Read the model definition and answer for the solid it produces. Units are mm, in the model's axes. Face numbers are marked on the shaded views. A direction names the side the tool comes from. Coordinates: 2 decimals unless noted, no trailing zeros. Write each loop counter-clockwise with the first axis right and the second up, starting at its lowest first coordinate (ties: lowest second). Pieces come first, ordered by that corner, then holes. Notation, with made-up numbers: (52.5, -37.75) - (64.5, -37.75) arc R25 cw to (64.5, -15.75) - close; hole circle Ø1 at (21, -28.75). An arc over 180 degrees is marked (long way). Use a Markdown table: item, result.
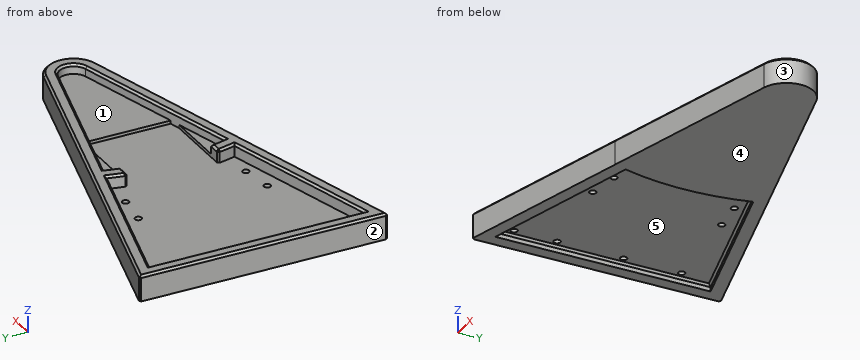
from build123d import *
from OCP.BRepFilletAPI import BRepFilletAPI_MakeChamfer

# Parameters (mm, degrees)
BOSS_EXTRUDE1_DEPTH     = 6
BOSS_EXTRUDE2_START     = 6
BOSS_EXTRUDE2_DEPTH     = 6
BOSS_EXTRUDE3_DEPTH     = 1.5
CUT_EXTRUDE3_DEPTH      = 6
CHAMFER1_SIZE           = 0.858848527
CHAMFER1_SIZE_2         = 1
CHAMFER2_SIZE           = 1
CHAMFER3_SIZE           = 1
CHAMFER3_SIZE2          = 0.816496581
CUT_EXTRUDE4_DEPTH      = 3
CHAMFER4_SIZE           = 1
CUT_EXTRUDE5_DEPTH      = 178.282114668
CUT_EXTRUDE5_DEPTH_BACK = 178.282114668
SKETCH8_R               = 1.55


with BuildPart() as part:
    # Sketch3 → Boss-Extrude1 (new body)
    with BuildSketch(Plane.XY):
        with BuildLine():
            Line((3.263957589, 12.181255556), (-167.389036276, 57.907587448))
            Line((-167.389036276, 57.907587448), (-167.389036276, -57.907587448))
            Line((-167.389036276, -57.907587448), (-83.597968128, -35.455838404))
            Line((-83.597968128, -35.455838404), (3.263957589, -12.181255556))
            ThreePointArc((3.263957589, -12.181255556), (12.610963724, 0), (3.263957589, 12.181255556))
        make_face()
    extrude(amount=BOSS_EXTRUDE1_DEPTH)

    # Sketch3<3> → Boss-Extrude2 (add)
    with BuildSketch(Plane.XY.offset(BOSS_EXTRUDE2_START)):
        with BuildLine():
            ThreePointArc((3.263957589, -12.181255556), (12.610963724, 0), (3.263957589, 12.181255556))
            Line((3.263957589, 12.181255556), (-167.389036276, 57.907587448))
            Line((-167.389036276, 57.907587448), (-167.389036276, -57.907587448))
            Line((-167.389036276, -57.907587448), (-83.597968128, -35.455838404))
            Line((-83.597968128, -35.455838404), (3.263957589, -12.181255556))
        make_face()
        with BuildLine():
            Line((1.711043318, -6.385700598), (-79.486479098, -28.142511157))
            ThreePointArc((-79.486479098, -28.142511157), (-83.143036276, 0), (-79.486479098, 28.142511157))
            Line((-79.486479098, 28.142511157), (1.711043318, 6.385700598))
            ThreePointArc((1.711043318, 6.385700598), (6.610963724, 0), (1.711043318, -6.385700598))
        make_face(mode=Mode.SUBTRACT)
        with BuildLine():
            Line((-85.282065581, -29.695433875), (-161.389036276, -50.088235211))
            Line((-161.389036276, -50.088235211), (-161.389036276, 50.088235211))
            Line((-161.389036276, 50.088235211), (-85.282065581, 29.695433875))
            ThreePointArc((-85.282065581, 29.695433875), (-89.143036276, 0), (-85.282065581, -29.695433875))
        make_face(mode=Mode.SUBTRACT)
    extrude(amount=BOSS_EXTRUDE2_DEPTH)

    # Sketch4 → Boss-Extrude3 (add)
    with BuildSketch(Plane.XY.offset(6)):
        with BuildLine():
            ThreePointArc((-79.486479098, 28.142511157), (-80.363791639, 24.584864194), (-81.12226241, 21))
            Line((-81.12226241, 21), (-52.830264568, 21))
            Line((-52.830264568, 21), (-79.486479098, 28.142511157))
        make_face()
        with BuildLine():
            Line((-79.486479098, -28.142511157), (-52.830264568, -21))
            Line((-52.830264568, -21), (-81.12226241, -21))
            ThreePointArc((-81.12226241, -21), (-80.363791639, -24.584864194), (-79.486479098, -28.142511157))
        make_face()
        with BuildLine():
            Line((-48.09821376, 19.732050808), (-48.09821376, -19.732050808))
            Line((-48.09821376, -19.732050808), (1.711043318, -6.385700598))
            ThreePointArc((1.711043318, -6.385700598), (6.610963724, 0), (1.711043318, 6.385700598))
            Line((1.711043318, 6.385700598), (-48.09821376, 19.732050808))
        make_face()
    extrude(amount=BOSS_EXTRUDE3_DEPTH)

    # Sketch5 → Cut-Extrude3 (cut)
    with BuildSketch(Plane.XY.offset(6)):
        with BuildLine():
            Line((-81.12226241, 21), (-87.228470489, 21))
            ThreePointArc((-87.228470489, 21), (-89.143036276, 0), (-87.228470489, -21))
            Line((-87.228470489, -21), (-81.12226241, -21))
            ThreePointArc((-81.12226241, -21), (-83.143036276, 0), (-81.12226241, 21))
        make_face()
    extrude(amount=CUT_EXTRUDE3_DEPTH, mode=Mode.SUBTRACT)

    # Chamfer1
    # the kernel refuses this chamfer: 1, 0.858848527 mm, written as the material it takes off along each edge
    with BuildSketch(Plane(origin=(-87.228470489, 21, 6), x_dir=(0.1850514416549976, 0.9827288354075131, 0), z_dir=(0, 0, 1))) as chamfer1_piece_1:
        with BuildLine():
            Line((0.995740125, 0), (CHAMFER1_SIZE * 0.185051441724, -CHAMFER1_SIZE * 0.982728835776))
            Line((CHAMFER1_SIZE * 0.185051441724, -CHAMFER1_SIZE * 0.982728835776), (0, 0))
            ThreePointArc((0, 0), (0.511949844, 0.001066408), (0.995740125, 0))
        make_face()
    extrude(amount=8.560742024, mode=Mode.SUBTRACT)
    with BuildSketch(Plane(origin=(-87.228470489, -21, 6), x_dir=(1, 0, 0), z_dir=(0, 0, 1))) as chamfer1_piece_2:
        with BuildLine():
            Line((CHAMFER1_SIZE_2, 0), (0.158025015, -0.841974985))
            ThreePointArc((0.158025015, -0.841974985), (0.080319075, -0.432228603), (0, 0))
            Line((0, 0), (CHAMFER1_SIZE_2, 0))
        make_face()
    extrude(amount=8.571682988, mode=Mode.SUBTRACT)

    # Chamfer2
    chamfer2_edges = [part.edges().sort_by_distance(p)[0] for p in [
        (-86.244364999, -25.784214234, 12),
        (-83.67536645, -21, 12),
        (-86.706914653, 21.489271267, 12),
        (-86.649457982, -21.420987493, 12),
        (-82.062539343, -35.044421502, 12),
        (12.610963724, 0, 12),
        (-161.389036276, 0, 12),
        (-86.228906055, 25.852006602, 12),
        (-123.335550929, -39.891834543, 12),
        (-38.88771789, 17.264105877, 12),
        (-38.88771789, -17.264105877, 12),
        (-82.062539343, 35.044421502, 12),
        (-167.389036276, 0, 12),
        (-123.335550929, 39.891834543, 12),
        (6.610963724, 0, 12),
        (-80.363791639, 24.584864194, 12),
        (-80.363791639, -24.584864194, 12),
        (-83.745942186, 21, 12),
    ]]
    chamfer(chamfer2_edges, length=CHAMFER2_SIZE)

    # Chamfer3: one chamfer whose edges measure the first distance from different faces: ONE call of the kernel's chamfer builder (chamfer() names one face for all edges)
    chamfer3_edges_1 = [part.edges().sort_by_distance(p)[0] for p in [
        (-167.389036276, -57.907587448, 5.5),
    ]]
    chamfer3_side_1 = [part.faces().sort_by_distance(p)[0] for p in [
        (-167.389036276, 0, 5.5),
    ]]
    chamfer3_edges_2 = [part.edges().sort_by_distance(p)[0] for p in [
        (-167.389036276, 57.907587448, 5.5),
    ]]
    chamfer3_side_2 = [part.faces().sort_by_distance(p)[0] for p in [
        (-82.062539343, 35.044421502, 5.5),
    ]]
    chamfer3 = BRepFilletAPI_MakeChamfer(part.part.solid().wrapped)
    for e in chamfer3_edges_1:
        chamfer3.Add(CHAMFER3_SIZE, CHAMFER3_SIZE2, e.wrapped, chamfer3_side_1[0].wrapped)  # the first distance lies on this face
    for e in chamfer3_edges_2:
        chamfer3.Add(CHAMFER3_SIZE, CHAMFER3_SIZE2, e.wrapped, chamfer3_side_2[0].wrapped)  # the first distance lies on this face
    add(Compound.cast(chamfer3.Shape()), mode=Mode.REPLACE)

    # Sketch7 → Cut-Extrude4 (cut)
    with BuildSketch(Plane(origin=(0, 0, 0), x_dir=(-1, 0, 0), z_dir=(0, 0, -1))):
        with BuildLine():
            Line((161.389036276, 50.088235211), (85.282065581, 29.695433875))
            ThreePointArc((85.282065581, 29.695433875), (89.143036276, 0), (85.282065581, -29.695433875))
            Line((85.282065581, -29.695433875), (161.389036276, -50.088235211))
            Line((161.389036276, -50.088235211), (161.389036276, 50.088235211))
        make_face()
    extrude(amount=-CUT_EXTRUDE4_DEPTH, mode=Mode.SUBTRACT)

    # Chamfer4
    chamfer4_edges = [part.edges().sort_by_distance(p)[0] for p in [
        (-89.143036276, 0, 3),
        (-123.335550929, 39.891834543, 3),
        (-161.389036276, 0, 3),
        (-123.335550929, -39.891834543, 3),
    ]]
    chamfer(chamfer4_edges, length=CHAMFER4_SIZE)

    # Sketch8 → Cut-Extrude5 (cut, two sides: drawn at the far end of the back side and taken through both)
    with BuildSketch(Plane(origin=(0, 0, 3), x_dir=(-1, 0, 0), z_dir=(0, 0, -1)).offset(-CUT_EXTRUDE5_DEPTH_BACK)):
        with Locations((157.889036276, 34.775263876)):
            Circle(SKETCH8_R)
        with Locations((157.889036276, 7.775263876)):
            Circle(SKETCH8_R)
        with Locations((157.889036276, -23.157763876)):
            Circle(SKETCH8_R)
        with Locations((157.889036276, -43.157763876)):
            Circle(SKETCH8_R)
        with Locations((98.643036276, 28)):
            Circle(SKETCH8_R)
        with Locations((113.643036276, 30)):
            Circle(SKETCH8_R)
        with Locations((98.643036276, -28)):
            Circle(SKETCH8_R)
        with Locations((113.643036276, -30)):
            Circle(SKETCH8_R)
    extrude(amount=CUT_EXTRUDE5_DEPTH + CUT_EXTRUDE5_DEPTH_BACK, mode=Mode.SUBTRACT)


solid = part.part
(1) A cutting plane is placed at B-B, the plane x = -126. Write down the section's boundary in (y, z).
Report:
| item | result |
|---|---|
| outline | (-46.82, 0) - (-40.61, 0) - (-40.61, 2) - (-39.57, 3) - (39.57, 3) - (40.61, 2) - (40.61, 0) - (46.82, 0) - (46.82, 11) - (45.78, 12) - (41.64, 12) - (40.61, 11) - (40.61, 6) - (-40.61, 6) - (-40.61, 11) - (-41.64, 12) - (-45.78, 12) - (-46.82, 11) - close |
(2) For the marked faces 1 and 2, determine the directions among +Z, -Z, +X, -X, +Y, -Y from which every point of the face is accessible in a straight line to the end or side of a thin tool.
Report:
| item | result |
|---|---|
| face 1 | +Z |
| face 2 | +Z, -Z, -X, +Y, -Y |
(3) Each of these flat-tipped pins is pushed along its axis until it touches: P1, Ø5, axis at x = -98.64, y = 28, coming from the +Z side; P2, Ø1.9, axis at x = -98.64, y = -28, coming from the -Z side; P3, Ø5.5, axis at x = -77, z = 9.5, coming from the +Y side; P4, Ø1.5, axis at x = -18.5, z = 3, coming from the +Y side. Where does it stop, or does it pass through?
Report:
| item | result |
|---|---|
| P1 | stops at z = 6 |
| P2 | passes through |
| P3 | stops at y = 34.42 |
| P4 | stops at y = 18.21 |
(4) A cutting plane is placed at A-A, the plane z = 9.25. Write down the section's boundary in (x, y), and give its area (3 significant figures).
Report:
| item | result |
|---|---|
| outline | (-167.39, -56.91) - (-166.6, -57.7) - (3.26, -12.18) arc R12.61 ccw to (3.26, 12.18) - (-166.42, 57.65) - (-167.39, 57.09) - close; hole (-161.39, -50.09) - (-85.28, -29.7) arc R116.13 cw to (-87.07, -21.84) - (-86.23, -21) - (-81.12, -21) arc R110.13 ccw to (-79.49, -28.14) - (1.71, -6.39) arc R6.61 ccw to (1.71, 6.39) - (-79.49, 28.14) arc R110.13 ccw to (-81.12, 21) - (-86.37, 21) - (-87.04, 21.98) arc R116.13 cw to (-85.28, 29.7) - (-161.39, 50.09) - close |
| area | 2,970 mm² |
(5) The mould has two halves that part along Y. Classify the marked faces 3, 4 and 5: pulls with the +Y half, pulls with the -Y half, needs draft (parallel to the pull), parting line crosses it, or undercut.
Report:
| item | result |
|---|---|
| face 3 | parting line crosses it |
| face 4 | needs draft |
| face 5 | undercut |
(6) A cutting plane is placed at C-C, the plane x = -65. Write down the section's boundary in (y, z).
Report:
| item | result |
|---|---|
| outline | (-30.47, 0) - (30.47, 0) - (30.47, 11) - (29.44, 12) - (25.3, 12) - (24.26, 11) - (24.26, 7.5) - (21, 7.5) - (21, 6) - (-21, 6) - (-21, 7.5) - (-24.26, 7.5) - (-24.26, 11) - (-25.3, 12) - (-29.44, 12) - (-30.47, 11) - close |
(7) Straight lines are drawn through the part: L1, parallel to Z at x = -83.5, y = -6.5; L2, parallel to Z at x = -88.5, y = -29.5; L3, parallel to Y at x = -92.5, z = 8.25. For each, find the intervals that lie inside material, in ascending order.
Report:
| item | result |
|---|---|
| L1 | z = 0 to 6 |
| L2 | z = 3 to 6 |
| L3 | y = -37.84 to -31.63, 31.63 to 37.84 |
